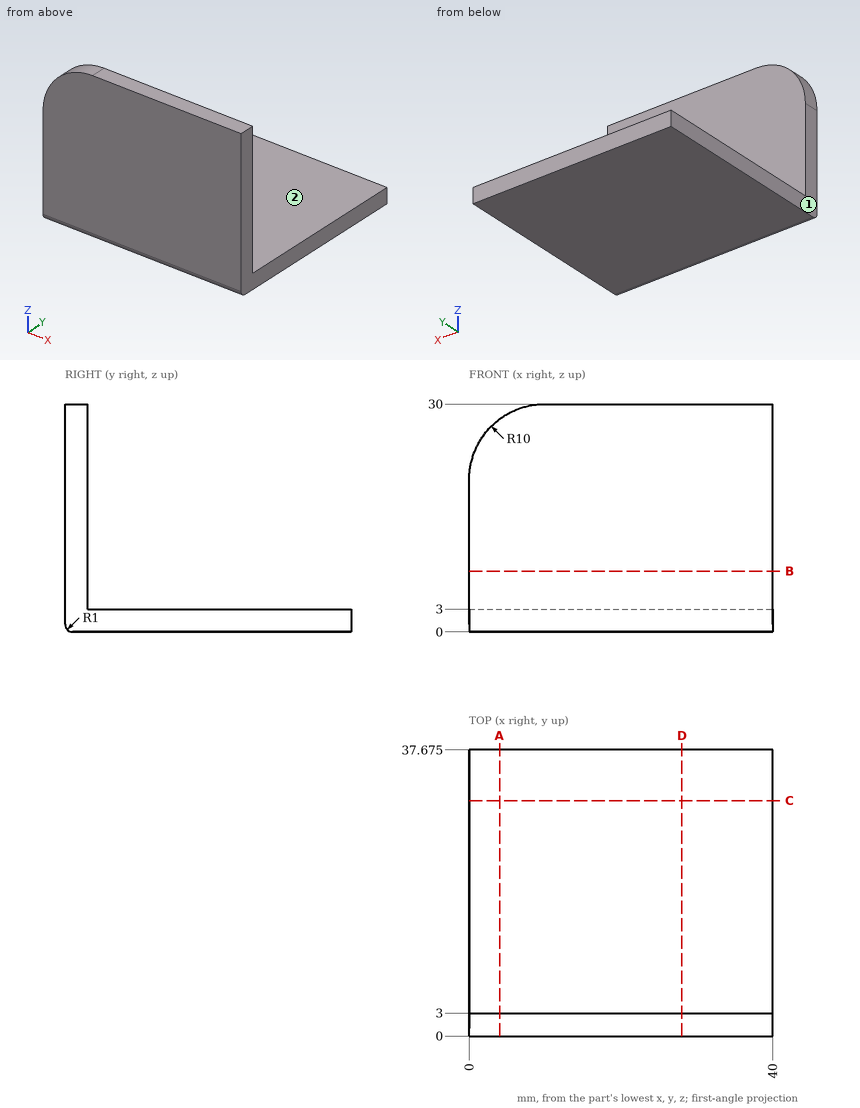
Input: dimensioned drawing with shaded views. Units: mm. Origin: part minimum x, y, z. A direction names the side the tool comes from. Round coordinates to 2 decimals unless told otherwise and drop trailing zeros. Loops run counter-clockwise (first coordinate to the right, second up) from the corner with the lowest first, then second, coordinate; pieces in that order, holes last. Notation, with made-up numbers: M 72,-40 L 89,-40 A23 cw 89,-18 Z; hole C -9.75,23.25 d3. An arc over 180 degrees is marked long. Return JSON: item names as keys, results as strings. Group by question number.
1. Material intervals for line 1 along Y through (x, z) = (26.5, 9.5), sorted ascending. Write a range as from..to.
2. Pin query (flat end, axial travel): pin 1 (13.5 mm diameter, centred on x = 15, z = 19.5, fed in from +Y). Return the tip coordinate at first contact, or that it passes through.
3. Reachability of the marked faces 1 and 2 from +Z, -Z, +X, -X, +Y, -Y: full face, straight path, thin tool, end or side. Return the list, or none.
4. Section query B-B on z = 8. Output: boundary loops of the cut face in (x, y).
5. Section query D-D on x = 28. Output: boundary loops of the cut face in (y, z) (1 decimal), and give its area (3 significant figures).
6. Section query A-A on x = 4. Output: boundary loops of the cut face in (y, z) (1 decimal).
Checks:
{
 "1": {"line 1": "y = 0..3"},
 "2": {"pin 1": "stops at y = 3"},
 "3": {"face 1": "+Z, -Z, -X, +Y, -Y", "face 2": "+Z, +X, -X, +Y"},
 "4": {"outline": "M 0,0 L 40,0 L 40,3 L 0,3 Z"},
 "5": {"outline": "M 0,1 A1 ccw 1,0 L 37.7,0 L 37.7,3 L 3,3 L 3,30 L 0,30 Z", "area": "194 mm²"},
 "6": {"outline": "M 0,1 A1 ccw 1,0 L 37.7,0 L 37.7,3 L 3,3 L 3,28 L 0,28 Z"}
}
